```python
from build123d import *

# Parameters (mm, degrees)
CROQUIS1_W              = 12
CROQUIS1_H              = 12
SALIENTE_EXTRUIR1_DEPTH = 20
CROQUIS2_W              = 12
CROQUIS2_H              = 1.5
CORTAR_EXTRUIR1_DEPTH   = 10
CROQUIS3_R              = 11.478178836
CROQUIS3_R_2            = 2
SALIENTE_EXTRUIR2_DEPTH = 3


with BuildPart() as part:
    # Croquis1 → Saliente-Extruir1 (new body)
    with BuildSketch(Plane(origin=(0, 0, 0), x_dir=(1, 0, 0), z_dir=(0, 1, 0))):
        with Locations((6, 6)):
            Rectangle(CROQUIS1_W, CROQUIS1_H)
    extrude(amount=SALIENTE_EXTRUIR1_DEPTH)

    # Croquis2 → Cortar-Extruir1 (cut)
    with BuildSketch(Plane.XY):
        with Locations((6, 17.25)):
            Rectangle(CROQUIS2_W, CROQUIS2_H)
    extrude(amount=-CORTAR_EXTRUIR1_DEPTH, mode=Mode.SUBTRACT)

    # Croquis3 → Saliente-Extruir2 (add)
    with BuildSketch(Plane.XZ):
        with Locations(Location((6, -6, 0), (0, 0, 270))):
            Circle(CROQUIS3_R)
        with Locations(Location((14.668474488, -6, 0), (0, 0, 270))):
            Circle(CROQUIS3_R_2, mode=Mode.SUBTRACT)
        with Locations(Location((6, -14.668474488, 0), (0, 0, 270))):
            Circle(CROQUIS3_R_2, mode=Mode.SUBTRACT)
        with Locations(Location((-2.668474488, -6, 0), (0, 0, 270))):
            Circle(CROQUIS3_R_2, mode=Mode.SUBTRACT)
        with Locations(Location((6, 2.668474488, 0), (0, 0, 270))):
            Circle(CROQUIS3_R_2, mode=Mode.SUBTRACT)
    extrude(amount=SALIENTE_EXTRUIR2_DEPTH)


solid = part.part
```
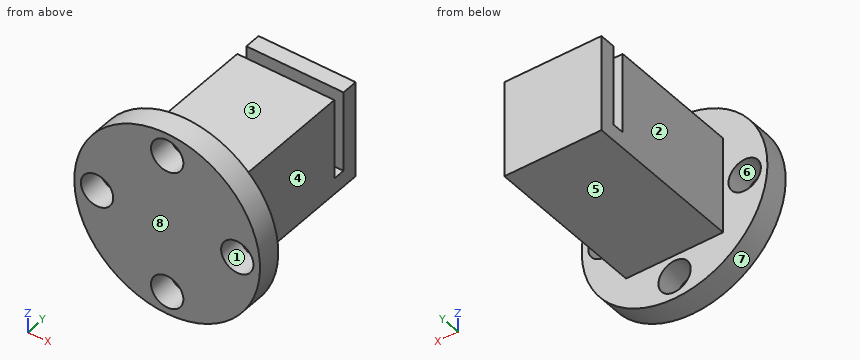
Verification items for the finished model (mm, model axes). Face numbers are marked on the shaded views. A direction names the side the tool comes from. Round coordinates to 2 decimals unless told otherwise and drop trailing zeros. Write each loop counter-clockwise with the first axis right and the second up, starting at its lowest first coordinate (ties: lowest second). Pieces come first, ordered by that corner, then holes. Notation, with made-up numbers: (48.25, 65) -> (69.25, 65) arc R26 ccw to (69.25, 97) -> close; hole circle Ø3 at (-28, 17). An arc over 180 degrees is marked (long way). Write each question's results on one line, items separated by ' | '.
Q1. Thickness scan on probe 1 along X at (y, z) = (-0.95, -6); probe 2 along Y at (x, z) = (1, -2.75); probe 3 along Y at (x, z) = (13.75, -10.25). Record the ranges inside material, lowest first.
Derived:
probe 1: x = -5.48 to -4.67, -0.67 to 12.67, 16.67 to 17.48 | probe 2: y = -3 to 16.5, 18 to 20 | probe 3: y = -3 to 0
Q2. Sectioned sample at B-B, the plane x = 6. Record the boundary of the cut face in (y, z), and give its area (3 significant figures).
Derived:
outline: (-3, -17.48) -> (0, -17.48) -> (0, -16.67) -> (-3, -16.67) -> close; (-3, -12.67) -> (0, -12.67) -> (0, -12) -> (20, -12) -> (20, 0) -> (18, 0) -> (18, -10) -> (16.5, -10) -> (16.5, 0) -> (0, 0) -> (0, 0.67) -> (-3, 0.67) -> close; (-3, 4.67) -> (0, 4.67) -> (0, 5.48) -> (-3, 5.48) -> close | area: 270 mm²
Q3. Sectioned sample at A-A, the plane z = -6. Record the boundary of the cut face in (x, y).
Derived:
outline: (-5.48, -3) -> (-4.67, -3) -> (-4.67, 0) -> (-5.48, 0) -> close; (-0.67, -3) -> (12.67, -3) -> (12.67, 0) -> (12, 0) -> (12, 16.5) -> (0, 16.5) -> (0, 0) -> (-0.67, 0) -> close; (0, 18) -> (12, 18) -> (12, 20) -> (0, 20) -> close; (16.67, -3) -> (17.48, -3) -> (17.48, 0) -> (16.67, 0) -> close
Q4. Sectioned sample at C-C, the plane x = -2. Record the boundary of the cut face in (y, z), and give its area (3 significant figures).
Derived:
outline: (-3, -14.23) -> (0, -14.23) -> (0, -7.88) -> (-3, -7.88) -> close; (-3, -4.12) -> (0, -4.12) -> (0, 2.23) -> (-3, 2.23) -> close | area: 38.1 mm²
Q5. Access from +Z, -Z, +X, -X, +Y, -Y to the whole of each face (thin tool, end or side, straight path). Record for the marked faces 1, 2, 3, 4 and 5.
Derived:
face 1: +Y, -Y | face 2: +Z, -Z, -X, +Y | face 3: +Z, +X, -X, +Y | face 4: +Z, -Z, +X, +Y | face 5: -Z, +X, -X, +Y
Q6. Draft check along X on the marked faces 6, 7 and 8. Enter one of: released by +X, released by -X, zero draft, split by the parting line, or undercut.
Derived:
face 6: undercut | face 7: split by the parting line | face 8: zero draft
Q7. Sectioned sample at D-D, the plane z = 1.5. Record the boundary of the cut face in (x, y).
Derived:
outline: (-2.69, -3) -> (4.38, -3) -> (4.38, 0) -> (-2.69, 0) -> close; (7.62, -3) -> (14.69, -3) -> (14.69, 0) -> (7.62, 0) -> close
Q8. Go/stop test with flat-tipped pins: pin 1 Ø4.5 at (x, z) = (6, 2.67) entering from +Y; pin 2 Ø1.2 at (x, y) = (6, 17.5) entering from +Z; pin 3 Ø6 at (y, z) = (5.5, -4.5) entering from +X. Record where each tip stops, or that it passes through.
Derived:
pin 1: stops at y = 0 | pin 2: stops at z = 0 | pin 3: stops at x = 12
